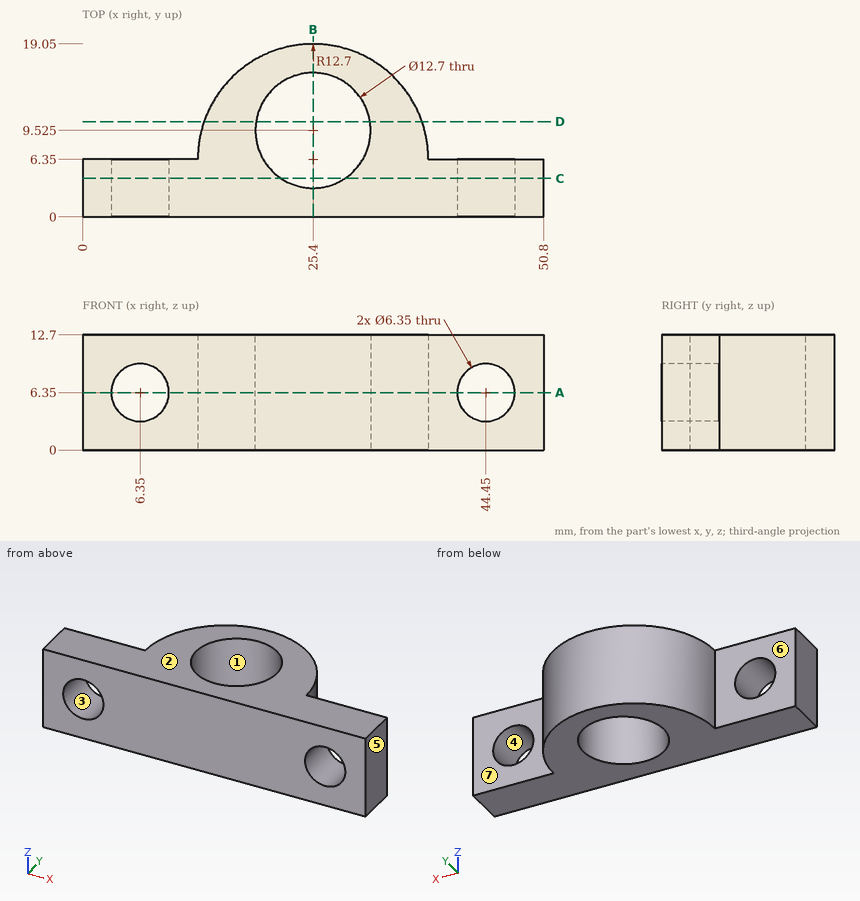
Verification items for this drawing (mm, ordinates from the low corner). A direction names the side the tool comes from. Give positions to 0.01 mm unless a question says otherwise; leave off trailing zeros. Loops run counter-clockwise (first coordinate to the right, second up) from the corner with the lowest first, then second, coordinate; pieces in that order, holes last. Notation, with made-up numbers: M 82.25,71 L 134.25,71 A25 cw 134.25,87 Z; hole C 41.5,58.25 d8. An arc over 180 degrees is marked long. Write item = value, one per line.
(1) Material ranges on line 1 (X direction, y = 1.75, z = 6.35) (3 decimals); line 2 (Z direction, x = 44.45, y = 2.75) (3 decimals); line 3 (X direction, y = 4, z = 6.35) (3 decimals), recorded low to high. Write a range as [from, to].
Answer below:
line_1 = [0, 3.175], [9.525, 41.275], [47.625, 50.8]
line_2 = [0, 3.175], [9.525, 12.7]
line_3 = [0, 3.175], [9.525, 22.27], [28.53, 41.275], [47.625, 50.8]
(2) Sectioned sample at C-C, the plane y = 4.25. Record the cut outline in (x, z) (3 decimals), plus the area to 3 significant figures.
Answer below:
outline = M 0,0 L 21.865,0 L 21.865,12.7 L 0,12.7 Z; M 28.935,0 L 50.8,0 L 50.8,12.7 L 28.935,12.7 Z; hole C 6.35,6.35 d6.35; hole C 44.45,6.35 d6.35
area = 492 mm2
(3) Sectioned sample at B-B, the plane x = 25.4. Record the cut outline in (y, z) (3 decimals).
Answer below:
outline = M 0,0 L 3.175,0 L 3.175,12.7 L 0,12.7 Z; M 15.875,0 L 19.05,0 L 19.05,12.7 L 15.875,12.7 Z
(4) Sectioned sample at D-D, the plane y = 10.5. Record the cut outline in (x, z).
Answer below:
outline = M 13.4,0 L 19.13,0 L 19.13,12.7 L 13.4,12.7 Z; M 31.67,0 L 37.4,0 L 37.4,12.7 L 31.67,12.7 Z
(5) Tool access check on the marked faces 5, 6 and 7. Record the directions out of +Z, -Z, +X, -X, +Y, -Y that give a thin tool (end or side, any length) a straight path to the whole face; none if there is none.
Answer below:
face_5 = +Z, -Z, +X, +Y, -Y
face_6 = +Z, -Z, -X, +Y
face_7 = +Z, -Z, +X, +Y
(6) Sectioned sample at A-A, the plane z = 6.35. Record the cut outline in (x, y) (3 decimals).
Answer below:
outline = M 0,0 L 3.175,0 L 3.175,6.35 L 0,6.35 Z; M 9.525,0 L 41.275,0 L 41.275,6.35 L 38.1,6.35 A12.7 ccw 12.7,6.35 L 9.525,6.35 Z; M 47.625,0 L 50.8,0 L 50.8,6.35 L 47.625,6.35 Z; hole C 25.4,9.525 d12.7
(7) Gauge pin test, flat ends, axial feed: pin 1 Ø4 at (x, z) = (38, 9.5) entering from +Y (3 decimals); pin 2 Ø1 at (x, z) = (23, 5.5) entering from +Y; pin 3 Ø2 at (y, z) = (5, 3) entering from -X. Record the tip position at first contact, or that the pin passes through.
Answer below:
pin_1 = 13.345
pin_2 = 18.91
pin_3 = 0
(8) Release check for a two-part mould opening along Z. For the marked faces 1, 2, 3 and 4 record: released by +Z, released by -Z, zero draft, split by the parting line, or undercut.
Answer below:
face_1 = zero draft
face_2 = released by +Z
face_3 = undercut
face_4 = undercut
